from build123d import *

# Parameters (mm, degrees)
EXTRUDE_1_DEPTH     = 15
FILLET_1_R          = 5
FILLET_2_R          = 5
FILLET_3_R          = 5
FILLET_4_R          = 5
FILLET_5_R          = 5
FILLET_6_R          = 5
FILLET_7_R          = 5
FILLET_8_R          = 5
FILLET_9_R          = 5
FILLET_10_R         = 5
FILLET_11_R         = 5
FILLET_12_R         = 5
FILLET_13_R         = 5
FILLET_14_R         = 5
FILLET_15_R         = 5
FILLET_16_R         = 5
SKETCH_5_R          = 1.5
CUT_EXTRUDE_1_DEPTH = 15


with BuildPart() as part:
    # 草图3 → 凸台-拉伸1 (new body)
    with BuildSketch(Plane.XY):
        with BuildLine():
            Line((101.99145665, -27.727634828), (114.18506552, -15.283623844))
            ThreePointArc((114.18506552, -15.283623844), (110, 0), (114.18506552, 15.283623844))
            Line((114.18506552, 15.283623844), (101.99145665, 27.727634828))
            Line((101.99145665, 27.727634828), (48.171786379, 31.57189699))
            Line((48.171786379, 31.57189699), (32.743622368, 18.278544642))
            ThreePointArc((32.743622368, 18.278544642), (37.5, 0), (32.743622368, -18.278544642))
            Line((32.743622368, -18.278544642), (48.171786379, -31.57189699))
            Line((48.171786379, -31.57189699), (101.99145665, -27.727634828))
        make_face()
        with BuildLine():
            ThreePointArc((42.839131819, -13.777110909), (45, 0), (42.839131819, 13.777110909))
            Line((42.839131819, 13.777110909), (51.574083604, 21.303398011))
            Line((51.574083604, 21.303398011), (97.500283316, 18.022955175))
            Line((97.500283316, 18.022955175), (106.212331228, 9.132000819))
            ThreePointArc((106.212331228, 9.132000819), (105, 0), (106.212331228, -9.132000819))
            Line((106.212331228, -9.132000819), (97.500283316, -18.022955175))
            Line((97.500283316, -18.022955175), (51.574083604, -21.303398011))
            Line((51.574083604, -21.303398011), (42.839131819, -13.777110909))
        make_face(mode=Mode.SUBTRACT)
    extrude(amount=EXTRUDE_1_DEPTH)

    # 圆角1
    fillet_1_edges = [part.edges().sort_by_distance(p)[0] for p in [
        (101.99145665, 27.727634828, 7.5),
    ]]
    fillet(fillet_1_edges, radius=FILLET_1_R)

    # 圆角2
    fillet_2_edges = [part.edges().sort_by_distance(p)[0] for p in [
        (114.18506552, 15.283623844, 7.5),
    ]]
    fillet(fillet_2_edges, radius=FILLET_2_R)

    # 圆角3
    fillet_3_edges = [part.edges().sort_by_distance(p)[0] for p in [
        (114.18506552, -15.283623844, 7.5),
    ]]
    fillet(fillet_3_edges, radius=FILLET_3_R)

    # 圆角4
    fillet_4_edges = [part.edges().sort_by_distance(p)[0] for p in [
        (101.99145665, -27.727634828, 7.5),
    ]]
    fillet(fillet_4_edges, radius=FILLET_4_R)

    # 圆角5
    fillet_5_edges = [part.edges().sort_by_distance(p)[0] for p in [
        (48.171786379, -31.57189699, 7.5),
    ]]
    fillet(fillet_5_edges, radius=FILLET_5_R)

    # 圆角6
    fillet_6_edges = [part.edges().sort_by_distance(p)[0] for p in [
        (48.171786379, 31.57189699, 7.5),
    ]]
    fillet(fillet_6_edges, radius=FILLET_6_R)

    # 圆角7
    fillet_7_edges = [part.edges().sort_by_distance(p)[0] for p in [
        (32.743622368, -18.278544642, 7.5),
    ]]
    fillet(fillet_7_edges, radius=FILLET_7_R)

    # 圆角8
    fillet_8_edges = [part.edges().sort_by_distance(p)[0] for p in [
        (32.743622368, 18.278544642, 7.5),
    ]]
    fillet(fillet_8_edges, radius=FILLET_8_R)

    # 圆角9
    fillet_9_edges = [part.edges().sort_by_distance(p)[0] for p in [
        (97.500283316, -18.022955175, 7.5),
    ]]
    fillet(fillet_9_edges, radius=FILLET_9_R)

    # 圆角10
    fillet_10_edges = [part.edges().sort_by_distance(p)[0] for p in [
        (106.212331228, -9.132000819, 7.5),
    ]]
    fillet(fillet_10_edges, radius=FILLET_10_R)

    # 圆角11
    fillet_11_edges = [part.edges().sort_by_distance(p)[0] for p in [
        (106.212331228, 9.132000819, 7.5),
    ]]
    fillet(fillet_11_edges, radius=FILLET_11_R)

    # 圆角12
    fillet_12_edges = [part.edges().sort_by_distance(p)[0] for p in [
        (97.500283316, 18.022955175, 7.5),
    ]]
    fillet(fillet_12_edges, radius=FILLET_12_R)

    # 圆角13
    fillet_13_edges = [part.edges().sort_by_distance(p)[0] for p in [
        (51.574083604, -21.303398011, 7.5),
    ]]
    fillet(fillet_13_edges, radius=FILLET_13_R)

    # 圆角14
    fillet_14_edges = [part.edges().sort_by_distance(p)[0] for p in [
        (42.839131819, -13.777110909, 7.5),
    ]]
    fillet(fillet_14_edges, radius=FILLET_14_R)

    # 圆角15
    fillet_15_edges = [part.edges().sort_by_distance(p)[0] for p in [
        (42.839131819, 13.777110909, 7.5),
    ]]
    fillet(fillet_15_edges, radius=FILLET_15_R)

    # 圆角16
    fillet_16_edges = [part.edges().sort_by_distance(p)[0] for p in [
        (51.574083604, 21.303398011, 7.5),
    ]]
    fillet(fillet_16_edges, radius=FILLET_16_R)

    # 草图5 → 切除-拉伸1 (cut)
    with BuildSketch(Plane(origin=(0, 0, 0), x_dir=(-1, 0, 0), z_dir=(0, 0, -1))):
        with Locations((-36.9551813, 15.307337295)):
            Circle(SKETCH_5_R)
        with Locations((-40, 0)):
            Circle(SKETCH_5_R)
        with Locations((-36.9551813, -15.307337295)):
            Circle(SKETCH_5_R)
        with Locations((-49.872934992, -26.437647501)):
            Circle(SKETCH_5_R)
        with Locations((-49.872934992, 26.437647501)):
            Circle(SKETCH_5_R)
        with Locations((-99.745869983, 22.875295001)):
            Circle(SKETCH_5_R)
        with Locations((-99.745869983, -22.875295001)):
            Circle(SKETCH_5_R)
        with Locations((-109.973915193, 12.437211552)):
            Circle(SKETCH_5_R)
        with Locations((-107.5, 0)):
            Circle(SKETCH_5_R)
        with Locations((-109.973915193, -12.437211552)):
            Circle(SKETCH_5_R)
        with Locations((-59.84752199, 25.725177001)):
            Circle(SKETCH_5_R)
        with Locations((-69.822108988, 25.012706501)):
            Circle(SKETCH_5_R)
        with Locations((-79.796695986, 24.300236001)):
            Circle(SKETCH_5_R)
        with Locations((-89.771282985, 23.587765501)):
            Circle(SKETCH_5_R)
        with Locations((-89.771282985, -23.587765501)):
            Circle(SKETCH_5_R)
        with Locations((-79.796695986, -24.300236001)):
            Circle(SKETCH_5_R)
        with Locations((-69.822108988, -25.012706501)):
            Circle(SKETCH_5_R)
        with Locations((-59.84752199, -25.725177001)):
            Circle(SKETCH_5_R)
    extrude(amount=-CUT_EXTRUDE_1_DEPTH, mode=Mode.SUBTRACT)


solid = part.part
Model file for the job. Use its own axes, mm. A direction names the side the tool comes from. Round coordinates to 2 decimals unless told otherwise and drop trailing zeros. Loops run counter-clockwise (first coordinate to the right, second up) from the corner with the lowest first, then second, coordinate; pieces in that order, holes last. Notation, with made-up numbers: M 18,46.25 L 39,46.25 A25 ccw 39,85.25 Z; hole C 21,76 d10. An arc over 180 degrees is marked long. One line per question, with ' | ' between items.
1) Drill centre lines: line 1 along X through (y, z) = (-12, 6.75); line 2 along X through (y, z) = (-25.5, 2); line 3 along X through (y, z) = (15, 3). Where is each one in solid material? Low to high.
Solved:
line 1: x = 35.53 to 43.52, 103.4 to 108.54, 111.41 to 112.5 | line 2: x = 41.12 to 48.7, 51.04 to 58.36, 61.33 to 68.4, 71.24 to 78.9, 80.7 to 104.17 | line 3: x = 34.37 to 35.49, 38.42 to 44.47, 100.46 to 113.04
2) Band-saw the part on D-D (x = 40). Give the cut face in (y, z).
Solved:
outline: M -24.53,0 L -1.5,0 L -1.5,15 L -24.53,15 Z; M 1.5,0 L 24.53,0 L 24.53,15 L 1.5,15 Z
3) Flat gauge pins, fed straight in: pin 1 (6 mm diameter, centred on y = -11.5, z = 12.5, fed in from -X); pin 2 (2.5 mm diameter, centred on x = 79.8, y = 24.3, fed in from +Z) (3 decimals); pin 3 (8 mm diameter, centred on y = 5.5, z = 12, fed in from -X); pin 4 (2 mm diameter, centred on y = -15.5, z = 12.5, fed in from -X). Where does each tip first touch, or does it go through?
Solved:
pin 1: stops at x = 34.58 | pin 2: passes through | pin 3: stops at x = 36.28 | pin 4: stops at x = 33.97
4) Band-saw the part on B-B (x = 64.5). Give the cut face in (y, z).
Solved:
outline: M -30.41,0 L -20.38,0 L -20.38,15 L -30.41,15 Z; M 20.38,0 L 30.41,0 L 30.41,15 L 20.38,15 Z
5) Mould opens along Y. For faces 1 (the cylindrical face through (48.326, -31.192, 7.605)), 2 (the flat face through (41.22, 25.58, 7.4)), 3 (the cylindrical face through (113.014, -15.201, 7.605)) say: +Y half, -Y half, draft (parallel to the pull), parting line (faces both ways), or undercut.
Solved:
face 1: -Y half | face 2: +Y half | face 3: undercut
6) Band-saw the part on C-C (z = 2.75). Give the number of separate pieces and of enclosed holes in the cut face, then the cut area to 3 significant figures.
Solved:
separate pieces: 1 | enclosed holes: 19 | area: 1,850 mm²
7) 3-axis set-ups, long thin cutter, end or side, ignore diameter. For faces 4 (the cylindrical face through (105.504, -9.06, 7.605)), 5 (the cylindrical face through (34.06, 18.09, 7.6)): which of +Z, -Z, +X, -X, +Y, -Y reach the whole face in a straight line?
Solved:
face 4: +Z, -Z | face 5: +Z, -Z, -X
8) Band-saw the part on A-A (y = 0). Give the cut face in (x, z).
Solved:
outline: M 37.5,0 L 38.5,0 L 38.5,15 L 37.5,15 Z; M 41.5,0 L 45,0 L 45,15 L 41.5,15 Z; M 105,0 L 106,0 L 106,15 L 105,15 Z; M 109,0 L 110,0 L 110,15 L 109,15 Z
